Geometry check sheet. Reference: the model listing, model coordinates, mm. A direction names the side the tool comes from. Give positions to 0.01 mm unless a question says otherwise; leave off trailing zeros. Loops run counter-clockwise (first coordinate to the right, second up) from the corner with the lowest first, then second, coordinate; pieces in that order, holes last. Notation, with made-up numbers: (-21.5, 86.5) -> (20.5, 86.5) arc R20 cw to (20.5, 116.5) -> close; hole circle Ø9 at (-37.75, -23.75). An arc over 180 degrees is marked (long way). Write item = value, one per line.
```python
from build123d import *

# Parameters (mm, degrees)
SKETCH_1_R          = 10
EXTRUDE_1_DEPTH     = 30
SKETCH_2_R          = 1.85
CUT_EXTRUDE_1_DEPTH = 34.166247904
SKETCH_3_R          = 1.85
SKETCH_3_R_2        = 1.6
EXTRUDE_2_DEPTH     = 15
CUT_EXTRUDE_START   = -15
SKETCH_4_R          = 2.5
SKETCH_4_R_2        = 1.85
CUT_EXTRUDE_2_DEPTH = 15
EXTRUDE_START       = -15
SKETCH_5_R          = 1.85
SKETCH_5_R_2        = 1.6
EXTRUDE_3_DEPTH     = 15
SKETCH_6_R          = 2.5
CUT_EXTRUDE_4_DEPTH = 15
SKETCH_8_W          = 25
SKETCH_8_H          = 25
SKETCH_8_R          = 10
EXTRUDE_4_DEPTH     = 3
FILLET_1_R          = 4
FILLET_6_R          = 12.5
FILLET_7_R          = 12.5
FILLET_8_R          = 12.5
FILLET_9_R          = 12.5
EXTRUDE_START_2     = -25
SKETCH_9_R          = 2.5
EXTRUDE_6_DEPTH     = 25
SKETCH_10_R         = 1.9
CUT_EXTRUDE_5_DEPTH = 10
SKETCH_11_R         = 3
CUT_EXTRUDE_6_DEPTH = 15


# Some blends are built 0.0001 mm under size
with BuildPart() as part:
    # 草图1 → 凸台-拉伸1 (new body)
    with BuildSketch(Plane(origin=(0, 0, 0), x_dir=(1, 0, 0), z_dir=(0, 1, 0))):
        with Locations(Location((0, 0, 0), (0, 0, 270))):
            Circle(SKETCH_1_R)
    extrude(amount=EXTRUDE_1_DEPTH)

    # 草图2 → 切除-拉伸1 (cut, through all)
    with BuildSketch(Plane(origin=(0, 30, 0), x_dir=(1, 0, 0), z_dir=(0, 1, 0))):
        with Locations(Location((0, 6, 0), (0, 0, 270))):
            Circle(SKETCH_2_R)
        with Locations(Location((5.196152423, 3, 0), (0, 0, 270))):
            Circle(SKETCH_2_R)
        with Locations(Location((5.196152423, -3, 0), (0, 0, 270))):
            Circle(SKETCH_2_R)
        with Locations(Location((0, -6, 0), (0, 0, 270))):
            Circle(SKETCH_2_R)
        with Locations(Location((-5.196152423, -3, 0), (0, 0, 270))):
            Circle(SKETCH_2_R)
        with Locations(Location((-5.196152423, 3, 0), (0, 0, 270))):
            Circle(SKETCH_2_R)
    extrude(amount=-CUT_EXTRUDE_1_DEPTH, mode=Mode.SUBTRACT)

    # 草图3 → 凸台-拉伸2 (add)
    # profile 1 of 3: a face of its own
    with BuildSketch(Plane(origin=(0, 30, 0), x_dir=(1, 0, 0), z_dir=(0, 1, 0))):
        with Locations(Location((0, 6, 0), (0, 0, 270))):
            Circle(SKETCH_3_R)
        with Locations(Location((0, 6, 0), (0, 0, 270))):
            Circle(SKETCH_3_R_2, mode=Mode.SUBTRACT)
    # profile 2 of 3: a face of its own
    with BuildSketch(Plane(origin=(0, 30, 0), x_dir=(1, 0, 0), z_dir=(0, 1, 0))):
        with Locations(Location((-5.196152423, -3, 0), (0, 0, 270))):
            Circle(SKETCH_3_R)
        with Locations(Location((-5.196152423, -3, 0), (0, 0, 270))):
            Circle(SKETCH_3_R_2, mode=Mode.SUBTRACT)
    # profile 3 of 3: a face of its own
    with BuildSketch(Plane(origin=(0, 30, 0), x_dir=(1, 0, 0), z_dir=(0, 1, 0))):
        with Locations(Location((5.196152423, -3, 0), (0, 0, 270))):
            Circle(SKETCH_3_R)
        with Locations(Location((5.196152423, -3, 0), (0, 0, 270))):
            Circle(SKETCH_3_R_2, mode=Mode.SUBTRACT)
    extrude(amount=-EXTRUDE_2_DEPTH)

    # 草图4 → 切除-拉伸2 (cut)
    # profile 1 of 3: a face of its own
    with BuildSketch(Plane.XZ.offset(CUT_EXTRUDE_START)):
        with Locations(Location((-5.196152423, 3, 0), (0, 0, 270))):
            Circle(SKETCH_4_R)
        with Locations((-5.196152423, 3)):
            Circle(SKETCH_4_R_2, mode=Mode.SUBTRACT)
    # profile 2 of 3: a face of its own
    with BuildSketch(Plane.XZ.offset(CUT_EXTRUDE_START)):
        with Locations(Location((5.196152423, 3, 0), (0, 0, 270))):
            Circle(SKETCH_4_R)
        with Locations((5.196152423, 3)):
            Circle(SKETCH_4_R_2, mode=Mode.SUBTRACT)
    # profile 3 of 3: a face of its own
    with BuildSketch(Plane.XZ.offset(CUT_EXTRUDE_START)):
        with Locations(Location((0, -6, 0), (0, 0, 270))):
            Circle(SKETCH_4_R)
        with Locations((0, -6)):
            Circle(SKETCH_4_R_2, mode=Mode.SUBTRACT)
    extrude(amount=CUT_EXTRUDE_2_DEPTH, mode=Mode.SUBTRACT)

    # 草图5 → 凸台-拉伸3 (add)
    # profile 1 of 3: a face of its own
    with BuildSketch(Plane.XZ.offset(EXTRUDE_START)):
        with Locations(Location((0, 6, 0), (0, 0, 90))):
            Circle(SKETCH_5_R)
        with Locations(Location((0, 6, 0), (0, 0, 270))):
            Circle(SKETCH_5_R_2, mode=Mode.SUBTRACT)
    # profile 2 of 3: a face of its own
    with BuildSketch(Plane.XZ.offset(EXTRUDE_START)):
        with Locations(Location((-5.196152423, -3, 0), (0, 0, 90))):
            Circle(SKETCH_5_R)
        with Locations(Location((-5.196152423, -3, 0), (0, 0, 270))):
            Circle(SKETCH_5_R_2, mode=Mode.SUBTRACT)
    # profile 3 of 3: a face of its own
    with BuildSketch(Plane.XZ.offset(EXTRUDE_START)):
        with Locations(Location((5.196152423, -3, 0), (0, 0, 90))):
            Circle(SKETCH_5_R)
        with Locations(Location((5.196152423, -3, 0), (0, 0, 270))):
            Circle(SKETCH_5_R_2, mode=Mode.SUBTRACT)
    extrude(amount=EXTRUDE_3_DEPTH)

    # 草图6 → 切除-拉伸4 (cut)
    with BuildSketch(Plane(origin=(0, 30, 0), x_dir=(1, 0, 0), z_dir=(0, 1, 0))):
        with Locations(Location((-5.196152423, 3, 0), (0, 0, 270))):
            Circle(SKETCH_6_R)
        with Locations(Location((5.196152423, 3, 0), (0, 0, 270))):
            Circle(SKETCH_6_R)
        with Locations(Location((0, -6, 0), (0, 0, 270))):
            Circle(SKETCH_6_R)
    extrude(amount=-CUT_EXTRUDE_4_DEPTH, mode=Mode.SUBTRACT)

    # 草图8 → 凸台-拉伸4 (add)
    with BuildSketch(Plane.XZ):
        Rectangle(SKETCH_8_W, SKETCH_8_H)
        with Locations(Location((0, 0, 0), (0, 0, 270))):
            Circle(SKETCH_8_R, mode=Mode.SUBTRACT)
    extrude(amount=-EXTRUDE_4_DEPTH)

    # 圆角1
    # the kernel refuses this fillet: 4 mm, written as the material it adds along each edge
    with BuildSketch(Plane(origin=(0, 3, 0), x_dir=(0, 0, 1), z_dir=(-1, 0, 0))) as fillet_1_piece_1_section:
        with BuildLine():
            CenterArc((10 + FILLET_1_R, FILLET_1_R), FILLET_1_R, 180, 90)
            Line((10 + FILLET_1_R, 0), (10, 0))
            Line((10, 0), (10, FILLET_1_R))
        make_face()
    fillet_1_piece_1 = revolve(axis=Axis((0, 3, 0), (0, 1, 0)), mode=Mode.PRIVATE)
    fillet_1_piece_1 = split(fillet_1_piece_1, bisect_by=Plane(origin=(-12.5, 4.125745955, -11.125745955), z_dir=(1, 0, 0)), keep=Keep.TOP, mode=Mode.PRIVATE)
    fillet_1_piece_1 = split(fillet_1_piece_1, bisect_by=Plane(origin=(0, 4.125745955, 12.5), z_dir=(0, 0, -1)), keep=Keep.TOP, mode=Mode.PRIVATE)
    fillet_1_piece_1 = split(fillet_1_piece_1, bisect_by=Plane(origin=(12.5, 4.125745955, -11.125745955), z_dir=(-1, 0, 0)), keep=Keep.TOP, mode=Mode.PRIVATE)
    fillet_1_piece_1 = split(fillet_1_piece_1, bisect_by=Plane(origin=(0, 4.125745955, -12.5), z_dir=(0, 0, 1)), keep=Keep.TOP, mode=Mode.PRIVATE)
    add(fillet_1_piece_1)

    # 圆角6
    fillet_6_edges = [part.edges().sort_by_distance(p)[0] for p in [
        (12.5, 1.5, 12.5),
    ]]
    fillet(fillet_6_edges, radius=FILLET_6_R)

    # 圆角7
    fillet_7_edges = [part.edges().sort_by_distance(p)[0] for p in [
        (-12.5, 1.5, 12.5),
    ]]
    fillet(fillet_7_edges, radius=FILLET_7_R - 0.0001)  # a hair under: the kernel refuses the full size

    # 圆角8
    fillet_8_edges = [part.edges().sort_by_distance(p)[0] for p in [
        (-12.5, 1.5, -12.5),
    ]]
    fillet(fillet_8_edges, radius=FILLET_8_R)

    # 圆角9
    fillet_9_edges = [part.edges().sort_by_distance(p)[0] for p in [
        (12.5, 1.5, -12.5),
    ]]
    fillet(fillet_9_edges, radius=FILLET_9_R - 0.0001)  # a hair under: the kernel refuses the full size

    # 草图9 → 凸台-拉伸6 (add)
    with BuildSketch(Plane.XZ.offset(EXTRUDE_START_2)):
        with Locations((5.196152423, 3)):
            Circle(SKETCH_9_R)
        with Locations((-5.196152423, 3)):
            Circle(SKETCH_9_R)
        with Locations((0, -6)):
            Circle(SKETCH_9_R)
    extrude(amount=EXTRUDE_6_DEPTH)

    # 草图10 → 切除-拉伸5 (cut)
    with BuildSketch(Plane(origin=(0, 30, 0), x_dir=(1, 0, 0), z_dir=(0, 1, 0))):
        with Locations(Location((0, 6, 0), (0, 0, 270))):
            Circle(SKETCH_10_R)
        with Locations(Location((-5.196152423, -3, 0), (0, 0, 270))):
            Circle(SKETCH_10_R)
        with Locations(Location((5.196152423, -3, 0), (0, 0, 270))):
            Circle(SKETCH_10_R)
    extrude(amount=-CUT_EXTRUDE_5_DEPTH, mode=Mode.SUBTRACT)

    # 草图11 → 切除-拉伸6 (cut)
    with BuildSketch(Plane(origin=(0, 30, 0), x_dir=(1, 0, 0), z_dir=(0, 1, 0))):
        with Locations(Location((-5.196152423, 3, 0), (0, 0, 270))):
            Circle(SKETCH_11_R)
        with Locations(Location((5.196152423, 3, 0), (0, 0, 270))):
            Circle(SKETCH_11_R)
        with Locations(Location((0, -6, 0), (0, 0, 270))):
            Circle(SKETCH_11_R)
    extrude(amount=-CUT_EXTRUDE_6_DEPTH, mode=Mode.SUBTRACT)


solid = part.part
```
Item 1: Section check A-A, the plane y = 25. Record the cut outline in (x, z).
Answer:
outline = circle Ø20 at (0, 0); hole circle Ø6 at (-5.2, -3); hole circle Ø3.8 at (-5.2, 3); hole circle Ø6 at (0, 6); hole circle Ø3.8 at (0, -6); hole circle Ø6 at (5.2, -3); hole circle Ø3.8 at (5.2, 3)
Item 2: Tool access check on faces 4 (the cylindrical face through (8.741, 1.669, 8.935)), 5 (the cylindrical face through (0.08, 25.07, -7.9)). Record the directions out of +Z, -Z, +X, -X, +Y, -Y that give a thin tool (end or side, any length) a straight path to the whole face; none if there is none.
Answer:
face_4 = +Z, +X, +Y, -Y
face_5 = +Y
Item 3: Section check C-C, the plane y = 14.5. Record the cut outline in (x, z), plus the area to 3 significant figures.
Answer:
outline = circle Ø20 at (0, 0); hole circle Ø3.2 at (-5.2, -3); hole circle Ø3.2 at (0, 6); hole circle Ø3.2 at (5.2, -3)
area = 290 mm^2
Item 4: Gauge pin test, flat ends, axial feed: pin 1 (12 mm diameter, centred on x = 8, y = 15.5, fed in from +Z); pin 2 (4 mm diameter, centred on y = 10, z = -0.5, fed in from +X); pin 3 (3 mm diameter, centred on x = -6, z = -4, fed in from +Y). Record the tip position at first contact, or that the pin passes through.
Answer:
pin_1 = 9.8
pin_2 = 10
pin_3 = 15
Item 5: Section check B-B, the plane z = -3. Give the number of separate pieces and of enclosed holes in the cut face, plus the area to 3 significant figures.
Answer:
separate_pieces = 3
enclosed_holes = 0
area = 319 mm^2
Item 6: Thickness scan on L1, parallel to Z at x = 4.5, y = 25.5; L2, parallel to Z at x = -2.75, y = 20.5; L3, parallel to X at y = 20.5, z = -3. Record the ranges inside material, lowest first. Write a range as [from, to].
Answer:
L1 = [-8.93, -5.92], [-0.08, 1.23], [4.77, 8.93]
L2 = [-9.61, -4.74], [-1.26, 4.8], [7.2, 9.61]
L3 = [-9.54, -8.2], [-2.2, 2.2], [8.2, 9.54]
Item 7: Draft check along X on faces 1 (the flat face through (0, 30, 0)), 2 (the cylindrical face through (-8.936, 1.669, 8.741)), 3 (the flat face through (1.3, 15, 7.3)). Enter one of: +X half, -X half, draft (parallel to the pull), parting line (faces both ways), or undercut.
Answer:
face_1 = draft
face_2 = -X half
face_3 = undercut
